```python
from build123d import *

# Parameters (mm, degrees)
SKETCH1_W                = 88.9
SKETCH1_H                = 152.4
SKETCH1_R                = 2.38125
BOSS_EXTRUDE1_DEPTH      = 9.652
F_5_16_24_TAPPED_HOLE1_D = 6.9088
F_12_24_TAPPED_HOLE1_D   = 4.4958


with BuildPart() as part:
    # Sketch1 → Boss-Extrude1 (new body)
    with BuildSketch(Plane(origin=(0, 0, 0), x_dir=(1, 0, 0), z_dir=(0, 1, 0))):
        Rectangle(SKETCH1_W, SKETCH1_H)
        with Locations(Location((0, 0, 0), (0, 0, 270))):
            Circle(SKETCH1_R, mode=Mode.SUBTRACT)
    extrude(amount=BOSS_EXTRUDE1_DEPTH)

    # 5/16-24 Tapped Hole1 (through all)
    with Locations(Plane(origin=(0, 9.652, 0), x_dir=(1, 0, 0), z_dir=(0, 1, 0))):
        with Locations((19.05, 63.5), (-19.05, 63.5), (-19.05, 38.1), (19.05, 38.1), (19.05, 12.7), (19.05, -12.7), (19.05, -38.1), (19.05, -63.5), (-19.05, 12.7), (-19.05, -12.7), (-19.05, -38.1), (-19.05, -63.5)):
            Hole(F_5_16_24_TAPPED_HOLE1_D / 2)

    # #12-24 Tapped Hole1 (through all)
    with Locations(Plane(origin=(0, 9.652, 0), x_dir=(1, 0, 0), z_dir=(0, 1, 0))):
        with Locations((-31.75, 0), (31.75, 0), (-31.75, 12.7), (-31.75, 25.4), (31.75, 25.4), (31.75, 12.7), (31.75, -12.7), (31.75, -25.4), (-31.75, -12.7), (-31.75, -25.4)):
            Hole(F_12_24_TAPPED_HOLE1_D / 2)


solid = part.part
```
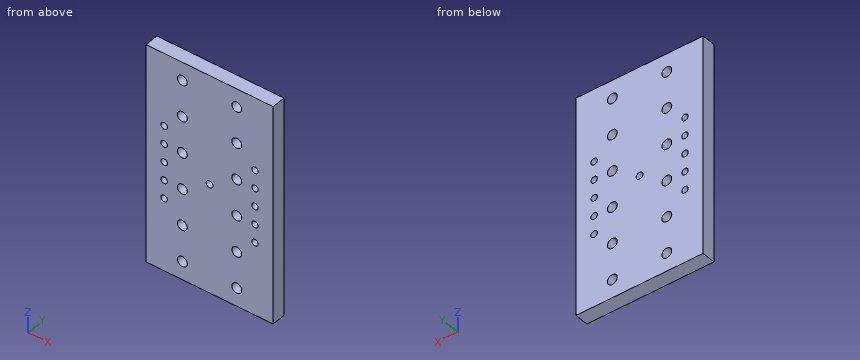
Model file for the job. Use its own axes, mm. Coordinates: 2 decimals unless noted, no trailing zeros. Order: outer loops, then holes, each group sorted by start corner. A loop starts at its lowest first (then second) coordinate and runs counter-clockwise, first axis right, second up. Notation, with made-up numbers: M -11.5,72 L 34.5,72 A12 ccw 34.5,89 Z; hole C 60.25,9.5 d7. An arc over 180 degrees is marked long. Answer as CSV lines item,"result".
(1) Band-saw the part on C-C, the plane y = 4. State how many separate pieces and enclosed holes the cut face has, then the cut area to 3 significant figures.
Geometry says:
separate pieces,"1"
enclosed holes,"23"
area,"12,900 mm2"
(2) Wall check: line 1 along X through (y, z) = (7.5, -38.1); line 2 along Z through (x, y) = (32, 6.5); line 3 along X through (y, z) = (4, 25.4). Give the ranges that are in metal, low to high.
Geometry says:
line 1,"x = -44.45 to -22.5, -15.6 to 15.6, 22.5 to 44.45"
line 2,"z = -76.2 to -27.63, -23.17 to -14.93, -10.47 to -2.23, 2.23 to 10.47, 14.93 to 23.17, 27.63 to 76.2"
line 3,"x = -44.45 to -34, -29.5 to 29.5, 34 to 44.45"
(3) Band-saw the part on B-B, the plane x = -31.75. List the corners of the cut face in (y, z), then the cut area to 3 significant figures.
Geometry says:
outline,"M 0,-76.2 L 9.65,-76.2 L 9.65,-27.65 L 0,-27.65 Z; M 0,-23.15 L 9.65,-23.15 L 9.65,-14.95 L 0,-14.95 Z; M 0,-10.45 L 9.65,-10.45 L 9.65,-2.25 L 0,-2.25 Z; M 0,2.25 L 9.65,2.25 L 9.65,10.45 L 0,10.45 Z; M 0,14.95 L 9.65,14.95 L 9.65,23.15 L 0,23.15 Z; M 0,27.65 L 9.65,27.65 L 9.65,76.2 L 0,76.2 Z"
area,"1,250 mm2"
(4) Band-saw the part on A-A, the plane z = 0. List the corners of the cut face in (x, y), then the cut area to 3 significant figures.
Geometry says:
outline,"M -44.45,0 L -34,0 L -34,9.65 L -44.45,9.65 Z; M -29.5,0 L -2.38,0 L -2.38,9.65 L -29.5,9.65 Z; M 2.38,0 L 29.5,0 L 29.5,9.65 L 2.38,9.65 Z; M 34,0 L 44.45,0 L 44.45,9.65 L 34,9.65 Z"
area,"725 mm2"
(5) Band-saw the part on D-D, the plane x = 19.05. List the corners of the cut face in (y, z), then the cut area to 3 significant figures.
Geometry says:
outline,"M 0,-76.2 L 9.65,-76.2 L 9.65,-66.95 L 0,-66.95 Z; M 0,-60.05 L 9.65,-60.05 L 9.65,-41.55 L 0,-41.55 Z; M 0,-34.65 L 9.65,-34.65 L 9.65,-16.15 L 0,-16.15 Z; M 0,-9.25 L 9.65,-9.25 L 9.65,9.25 L 0,9.25 Z; M 0,16.15 L 9.65,16.15 L 9.65,34.65 L 0,34.65 Z; M 0,41.55 L 9.65,41.55 L 9.65,60.05 L 0,60.05 Z; M 0,66.95 L 9.65,66.95 L 9.65,76.2 L 0,76.2 Z"
area,"1,070 mm2"
